from build123d import *

# Parameters (mm, degrees)
BOSS_EXTRUDE1_DEPTH                             = 10
BOSS_EXTRUDE2_DEPTH                             = 10
SKETCH4_R                                       = 2.4
CUT_EXTRUDE1_DEPTH                              = 8
SKETCH5_R                                       = 2.4
BOSS_EXTRUDE3_DEPTH                             = 12
CSK_FOR_M4_FLAT_HEAD_MACHINE_SCREW1_D           = 4.5
CSK_FOR_M4_FLAT_HEAD_MACHINE_SCREW1_DEPTH       = 10
CSK_FOR_M4_FLAT_HEAD_MACHINE_SCREW1_CSINK_D     = 9.4
CSK_FOR_M4_FLAT_HEAD_MACHINE_SCREW1_CSINK_ANGLE = 90
SKETCH10_R                                      = 2.4
BOSS_EXTRUDE4_DEPTH                             = 8
SKETCH11_R                                      = 4
BOSS_EXTRUDE5_DEPTH                             = 12
SKETCH12_R                                      = 4
BOSS_EXTRUDE6_DEPTH                             = 4


with BuildPart() as part:
    # Sketch2 → Boss-Extrude1 (new body)
    with BuildSketch(Plane(origin=(0, 0, 0), x_dir=(1, 0, 0), z_dir=(0, 1, 0))):
        Polygon((-64.864315762, -10.473994627), (-34.864315762, -10.473994627), (35.135684238, -10.473994627), (65.135684238, -10.473994627), (65.135684238, 23.526005373), (35.135684238, 23.526005373), (-34.864315762, 23.526005373), (-64.864315762, 23.526005373), align=None)
    extrude(amount=BOSS_EXTRUDE1_DEPTH)

    # Sketch3 → Boss-Extrude2 (add)
    with BuildSketch(Plane.XZ):
        Polygon((-34.864315762, 10.473994627), (-17.766011303, 10.473994627), (-17.766011303, 10.772744439), (-17.766011303, 12.772744439), (-17.766011303, 30.672744439), (-36.864315762, 30.672744439), (-56.864315762, 10.473994627), align=None)
        Polygon((-17.766011303, 10.772744439), (-17.766011303, 10.473994627), (35.135684238, 10.473994627), (57.135684238, 10.473994627), (37.135684238, 30.672744439), (-17.766011303, 30.672744439), (-17.766011303, 12.772744439), align=None)
    extrude(amount=-BOSS_EXTRUDE2_DEPTH)

    # Sketch4 → Cut-Extrude1 (cut)
    with BuildSketch(Plane(origin=(0, 10, 0), x_dir=(1, 0, 0), z_dir=(0, 1, 0))):
        with Locations((5.733988697, -27.172744439)):
            Circle(SKETCH4_R)
        with Locations((21.733988697, -27.172744439)):
            Circle(SKETCH4_R)
    extrude(amount=-CUT_EXTRUDE1_DEPTH, mode=Mode.SUBTRACT)

    # Sketch5 → Boss-Extrude3 (add)
    with BuildSketch(Plane(origin=(0, 10, 0), x_dir=(1, 0, 0), z_dir=(0, 1, 0))):
        with BuildLine():
            Line((42.233988697, -7.572744439), (65.333988697, -7.672744439))
            Line((65.333988697, -7.672744439), (65.333988697, -3.172744439))
            ThreePointArc((65.333988697, -3.172744439), (64.279573109, -0.627160027), (61.733988697, 0.427255561))
            Line((61.733988697, 0.427255561), (61.733988697, 0.327255561))
            Line((61.733988697, 0.327255561), (45.733988697, 0.327255561))
            ThreePointArc((45.733988697, 0.327255561), (43.259114963, -0.697870705), (42.233988697, -3.172744439))
            Line((42.233988697, -3.172744439), (42.233988697, -7.572744439))
        make_face()
        with Locations((61.733988697, -3.172744439)):
            Circle(SKETCH5_R, mode=Mode.SUBTRACT)
        with Locations((45.733988697, -3.172744439)):
            Circle(SKETCH5_R, mode=Mode.SUBTRACT)
    extrude(amount=BOSS_EXTRUDE3_DEPTH)

    # CSK for M4 Flat Head Machine Screw1
    with Locations(Plane(origin=(0, 10, 0), x_dir=(1, 0, 0), z_dir=(0, 1, 0))):
        with Locations((-58.864315762, 18.526005373), (-40.864315762, 18.526005373), (-58.864315762, -5.473994627), (-40.864315762, -5.473994627), (41.135684238, 18.526005373), (59.135684238, 18.526005373)):
            CounterSinkHole(CSK_FOR_M4_FLAT_HEAD_MACHINE_SCREW1_D / 2, CSK_FOR_M4_FLAT_HEAD_MACHINE_SCREW1_CSINK_D / 2, depth=CSK_FOR_M4_FLAT_HEAD_MACHINE_SCREW1_DEPTH, counter_sink_angle=CSK_FOR_M4_FLAT_HEAD_MACHINE_SCREW1_CSINK_ANGLE)

    # Sketch10 → Boss-Extrude4 (add)
    with BuildSketch(Plane(origin=(0, 10, 0), x_dir=(1, 0, 0), z_dir=(0, 1, 0))):
        with BuildLine():
            Line((-25.366011303, -16.042744439), (-9.366011303, -16.042744439))
            ThreePointArc((-9.366011303, -16.042744439), (-6.266011303, -19.142744439), (-9.366011303, -22.242744439))
            Line((-9.366011303, -22.242744439), (-25.366011303, -22.242744439))
            ThreePointArc((-25.366011303, -22.242744439), (-28.466011303, -19.142744439), (-25.366011303, -16.042744439))
        make_face()
        with Locations((-25.366011303, -19.142744439)):
            Circle(SKETCH10_R, mode=Mode.SUBTRACT)
        with Locations((-17.366011303, -19.142744439)):
            Circle(SKETCH10_R, mode=Mode.SUBTRACT)
        with Locations((-9.366011303, -19.142744439)):
            Circle(SKETCH10_R, mode=Mode.SUBTRACT)
        with BuildLine():
            Line((-25.366011303, 9.697255561), (-9.366011303, 9.697255561))
            ThreePointArc((-9.366011303, 9.697255561), (-6.266011303, 12.797255561), (-9.366011303, 15.897255561))
            Line((-9.366011303, 15.897255561), (-25.366011303, 15.897255561))
            ThreePointArc((-25.366011303, 15.897255561), (-28.466011303, 12.797255561), (-25.366011303, 9.697255561))
        make_face()
        with Locations((-9.366011303, 12.797255561)):
            Circle(SKETCH10_R, mode=Mode.SUBTRACT)
        with Locations((-17.366011303, 12.797255561)):
            Circle(SKETCH10_R, mode=Mode.SUBTRACT)
        with Locations((-25.366011303, 12.797255561)):
            Circle(SKETCH10_R, mode=Mode.SUBTRACT)
    extrude(amount=BOSS_EXTRUDE4_DEPTH)

    # Sketch11 → Boss-Extrude5 (add)
    with BuildSketch(Plane(origin=(0, 0, -13.526005373), x_dir=(-1, 0, 0), z_dir=(0, 0, -1))):
        with BuildLine():
            Line((-65.135684238, 10), (-35.135684238, 10))
            ThreePointArc((-35.135684238, 10), (-50.135684238, 25), (-65.135684238, 10))
        make_face()
        with Locations((-50.135684238, 16.7)):
            Circle(SKETCH11_R, mode=Mode.SUBTRACT)
    boss_extrude5 = extrude(amount=-BOSS_EXTRUDE5_DEPTH)

    # Sketch12 → Boss-Extrude6 (add)
    with BuildSketch(Plane.XY.offset(-1.526005373)):
        with Locations((50.135684238, 16.7)):
            Circle(SKETCH12_R)
    boss_extrude6 = extrude(amount=-BOSS_EXTRUDE6_DEPTH)

    # Mirror1: Boss-Extrude5, Boss-Extrude6 across plane
    add(boss_extrude5.mirror(Plane(origin=(0.135684238, 0, 0), x_dir=(0, 0, 1), z_dir=(1, 0, 0))))
    add(boss_extrude6.mirror(Plane(origin=(0.135684238, 0, 0), x_dir=(0, 0, 1), z_dir=(1, 0, 0))))


solid = part.part
Check sheet for the modelled part. Datum: model origin and axes. Units: mm. A direction names the side the tool comes from. Round coordinates to 2 decimals unless told otherwise and drop trailing zeros. Order: outer loops, then holes, each group sorted by start corner. A loop starts at its lowest first (then second) coordinate and runs counter-clockwise, first axis right, second up.
(1) Cross-section at C-C, the plane z = 14.5. Enter the section's corners in (x, y), and give its area (3 significant figures).
(2) Go/stop test with flat-tipped pins: P1, Ø5.5, axis at x = 21, z = 28, coming from the +Y side; P2, Ø6.5, axis at x = -51.5, y = 18, coming from the -Z side; P3, Ø2, axis at y = 14.5, z = 6, coming from the -X side. Record where each tip stops, or that it passes through.
(3) Cross-section at B-B, the plane x = 6.5. Enter the section's corners in (y, z).
(4) Cross-section at A-A, the plane y = 19.25. Enter the section's corners in (x, z).
(5) Scan lines: probe 1 along X at (y, z) = (21.75, 3); probe 2 along Y at (x, z) = (21, 1); probe 3 along X at (y, z) = (3.5, -20). Record each from-to range of solid material in increasing order.
(6) Cross-section at D-D, the plane x = 28. Enter the section's corners in (y, z).
(7) Access from +Z, -Z, +X, -X, +Y, -Y to the whole of each face (thin tool, end or side, straight path). Record for faces 5 (the flat face through (-17, 14, 22.243)), 6 (the flat face through (-53.4, 14.3, -13.526)), 7 (the flat face through (-17, 10, 19)), 8 (the cylindrical face through (-6.267, 13.944, 19.075)).
(8) Draft check along Z on faces 1 (the cylindrical face through (50, 25, -8)), 2 (the flat face through (50, 17, -5.526)), 3 (the flat face through (-46.724, 4.93, 20.715)), 4 (the flat face through (50, 16, -1.526)). Enter one of: pulls with the +Z half, pulls with the -Z half, needs draft (parallel to the pull), parting line crosses it, or undercut.
Check sheet entries:
1. outline: (-52.88, 0) - (53.15, 0) - (53.15, 10) - (-52.88, 10) - close
1. area: 1,060 mm2
2. P1: stops at y = 10
2. P2: stops at z = -13.53
2. P3: stops at x = 42.23
3. outline: (0, -23.53) - (10, -23.53) - (10, 24.9) - (2, 24.9) - (2, 29.45) - (10, 29.45) - (10, 30.67) - (0, 30.67) - close
4. outline: (-61.67, -13.53) - (-52.95, -13.53) - (-52.95, -5.53) - (-46.78, -5.53) - (-46.78, -13.53) - (-38.06, -13.53) - (-38.06, -1.53) - (-61.67, -1.53) - close; (38.33, -13.53) - (47.05, -13.53) - (47.05, -5.53) - (53.22, -5.53) - (53.22, -13.53) - (61.94, -13.53) - (61.94, -1.53) - (38.33, -1.53) - close; (42.23, 3.17) arc R3.5 ccw to (45.73, -0.33) - (61.73, -0.33) - (61.73, -0.43) arc R3.6 ccw to (65.33, 3.17) - (65.33, 7.67) - (42.23, 7.57) - close; hole circle Ø4.8 at (45.73, 3.17); hole circle Ø4.8 at (61.73, 3.17)
5. probe 1: x = 42.24 to 43.34, 48.13 to 59.34, 64.13 to 65.33
5. probe 2: y = 0 to 10
5. probe 3: x = -64.86 to -60.56, -57.16 to -42.56, -39.16 to 39.44, 42.84 to 57.44, 60.84 to 65.14
6. outline: (0, -23.53) - (10, -23.53) - (10, 30.67) - (0, 30.67) - close
7. face 5: +Z, +X, -X, +Y
7. face 6: -Z, -X, +Y
7. face 7: +Y
7. face 8: +X, +Y
8. face 1: needs draft
8. face 2: pulls with the -Z half
8. face 3: pulls with the +Z half
8. face 4: undercut
